Can you work these out from the model? Positions are in its coordinate system, mm. Face numbers are marked on the shaded views. A direction names the side the tool comes from. Give positions to 0.01 mm unless a question says otherwise; leave off trailing zeros. Loops run counter-clockwise (first coordinate to the right, second up) from the corner with the lowest first, then second, coordinate; pieces in that order, holes last. Notation, with made-up numbers: (-7.75, 76) -> (27.25, 76) arc R17 ccw to (27.25, 102) -> close; hole circle Ø10 at (56.25, 46.25). An arc over 180 degrees is marked (long way). One line per question, with ' | ' between items.
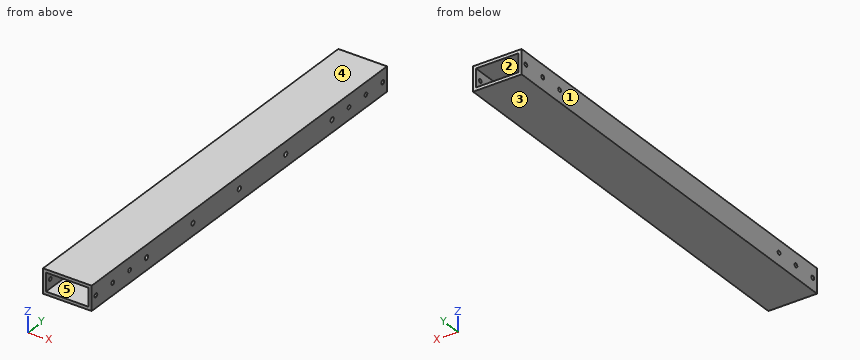
from build123d import *

# Parameters (mm, degrees)
SKETCH1_W           = 50.8
SKETCH1_H           = 25.4
SKETCH1_W_2         = 44.45
SKETCH1_H_2         = 19.05
BOSS_EXTRUDE1_DEPTH = 444.5
CUT_EXTRUDE1_REACH  = 412.536
SKETCH2_R           = 2.0828
SKETCH3_R           = 2.4257
CUT_EXTRUDE2_DEPTH  = 3.175


with BuildPart() as part:
    # Sketch1 → Boss-Extrude1 (new body)
    with BuildSketch(Plane(origin=(0, 0, 0), x_dir=(1, 0, 0), z_dir=(0, 1, 0))):
        with Locations((25.4, 12.7)):
            Rectangle(SKETCH1_W, SKETCH1_H)
        with Locations((25.4, 12.7)):
            Rectangle(SKETCH1_W_2, SKETCH1_H_2, mode=Mode.SUBTRACT)
    extrude(amount=BOSS_EXTRUDE1_DEPTH)

    # Cut-Extrude1: up to this face of the body (flat: up to its plane)
    cut_extrude1_end = Plane(part.part.faces().sort_by_distance((0, 222.25, -12.7))[0])
    # Sketch2 → Cut-Extrude1 (cut, up to the picked face)
    with BuildSketch(Plane(origin=(50.8, 398.917681448, 57.205629331), x_dir=(0, 0, 1), z_dir=(1, 0, 0)), mode=Mode.PRIVATE) as cut_extrude1_sk1:
        with Locations(Location((-69.905629331, -39.232318552, 0), (0, 0, 180))):
            Circle(SKETCH2_R)
    cut_extrude1_tool1 = split(extrude(cut_extrude1_sk1.sketch, amount=-CUT_EXTRUDE1_REACH, mode=Mode.PRIVATE), bisect_by=cut_extrude1_end, keep=Keep.BOTH, mode=Mode.PRIVATE)
    # Sketch2 → Cut-Extrude1 (cut, up to the picked face)
    with BuildSketch(Plane(origin=(50.8, 398.917681448, 57.205629331), x_dir=(0, 0, 1), z_dir=(1, 0, 0)), mode=Mode.PRIVATE) as cut_extrude1_sk2:
        with Locations(Location((-69.905629331, -13.832318552, 0), (0, 0, 180))):
            Circle(SKETCH2_R)
    cut_extrude1_tool2 = split(extrude(cut_extrude1_sk2.sketch, amount=-CUT_EXTRUDE1_REACH, mode=Mode.PRIVATE), bisect_by=cut_extrude1_end, keep=Keep.BOTH, mode=Mode.PRIVATE)
    # Sketch2 → Cut-Extrude1 (cut, up to the picked face)
    with BuildSketch(Plane(origin=(50.8, 398.917681448, 57.205629331), x_dir=(0, 0, 1), z_dir=(1, 0, 0)), mode=Mode.PRIVATE) as cut_extrude1_sk3:
        with Locations(Location((-69.905629331, 11.567681448, 0), (0, 0, 180))):
            Circle(SKETCH2_R)
    cut_extrude1_tool3 = split(extrude(cut_extrude1_sk3.sketch, amount=-CUT_EXTRUDE1_REACH, mode=Mode.PRIVATE), bisect_by=cut_extrude1_end, keep=Keep.BOTH, mode=Mode.PRIVATE)
    # Sketch2 → Cut-Extrude1 (cut, up to the picked face)
    with BuildSketch(Plane(origin=(50.8, 398.917681448, 57.205629331), x_dir=(0, 0, 1), z_dir=(1, 0, 0)), mode=Mode.PRIVATE) as cut_extrude1_sk4:
        with Locations(Location((-69.905629331, 341.767681448, 0), (0, 0, 180))):
            Circle(SKETCH2_R)
    cut_extrude1_tool4 = split(extrude(cut_extrude1_sk4.sketch, amount=-CUT_EXTRUDE1_REACH, mode=Mode.PRIVATE), bisect_by=cut_extrude1_end, keep=Keep.BOTH, mode=Mode.PRIVATE)
    # Sketch2 → Cut-Extrude1 (cut, up to the picked face)
    with BuildSketch(Plane(origin=(50.8, 398.917681448, 57.205629331), x_dir=(0, 0, 1), z_dir=(1, 0, 0)), mode=Mode.PRIVATE) as cut_extrude1_sk5:
        with Locations(Location((-69.905629331, 367.167681448, 0), (0, 0, 180))):
            Circle(SKETCH2_R)
    cut_extrude1_tool5 = split(extrude(cut_extrude1_sk5.sketch, amount=-CUT_EXTRUDE1_REACH, mode=Mode.PRIVATE), bisect_by=cut_extrude1_end, keep=Keep.BOTH, mode=Mode.PRIVATE)
    # Sketch2 → Cut-Extrude1 (cut, up to the picked face)
    with BuildSketch(Plane(origin=(50.8, 398.917681448, 57.205629331), x_dir=(0, 0, 1), z_dir=(1, 0, 0)), mode=Mode.PRIVATE) as cut_extrude1_sk6:
        with Locations(Location((-69.905629331, 392.567681448, 0), (0, 0, 180))):
            Circle(SKETCH2_R)
    cut_extrude1_tool6 = split(extrude(cut_extrude1_sk6.sketch, amount=-CUT_EXTRUDE1_REACH, mode=Mode.PRIVATE), bisect_by=cut_extrude1_end, keep=Keep.BOTH, mode=Mode.PRIVATE)
    add(cut_extrude1_tool1.solids().sort_by(Axis((50.8, 438.15, -12.7), (-1, 0, 0)))[0], mode=Mode.SUBTRACT)
    add(cut_extrude1_tool2.solids().sort_by(Axis((50.8, 412.75, -12.7), (-1, 0, 0)))[0], mode=Mode.SUBTRACT)
    add(cut_extrude1_tool3.solids().sort_by(Axis((50.8, 387.35, -12.7), (-1, 0, 0)))[0], mode=Mode.SUBTRACT)
    add(cut_extrude1_tool4.solids().sort_by(Axis((50.8, 57.15, -12.7), (-1, 0, 0)))[0], mode=Mode.SUBTRACT)
    add(cut_extrude1_tool5.solids().sort_by(Axis((50.8, 31.75, -12.7), (-1, 0, 0)))[0], mode=Mode.SUBTRACT)
    add(cut_extrude1_tool6.solids().sort_by(Axis((50.8, 6.35, -12.7), (-1, 0, 0)))[0], mode=Mode.SUBTRACT)

    # Sketch3 → Cut-Extrude2 (cut)
    with BuildSketch(Plane(origin=(50.8, 398.917681448, 57.205629331), x_dir=(0, 0, 1), z_dir=(1, 0, 0))):
        with Locations(Location((-69.905629331, 36.967681448, 0), (0, 0, 180))):
            Circle(SKETCH3_R)
        with Locations(Location((-69.905629331, 106.817681448, 0), (0, 0, 180))):
            Circle(SKETCH3_R)
        with Locations(Location((-69.905629331, 176.667681448, 0), (0, 0, 180))):
            Circle(SKETCH3_R)
        with Locations(Location((-69.905629331, 246.517681448, 0), (0, 0, 180))):
            Circle(SKETCH3_R)
        with Locations(Location((-69.905629331, 316.367681448, 0), (0, 0, 180))):
            Circle(SKETCH3_R)
    extrude(amount=-CUT_EXTRUDE2_DEPTH, mode=Mode.SUBTRACT)


solid = part.part
Q1. If we section it at A-A (x = 31): Write out the boundary of the cut face in (y, z) (3 decimals), plus the area to 3 significant figures.
Entries:
outline: (0, -25.4) -> (444.5, -25.4) -> (444.5, -22.225) -> (0, -22.225) -> close; (0, -3.175) -> (444.5, -3.175) -> (444.5, 0) -> (0, 0) -> close | area: 2,820 mm²
Q2. If we mould it in two halves opening along Z, with no side actions, what happens to the marked faces 1, 2 and 3? For each: pulls with the +Z half, pulls with the -Z half, needs draft (parallel to the pull), parting line crosses it, or undercut.
Entries:
face 1: needs draft | face 2: undercut | face 3: pulls with the -Z half
Q3. On a 3-axis mill with a long thin cutter (end or side, diameter ignored), from which of +Z, -Z, +X, -X, +Y, -Y can I reach the whole of each face in a straight line? I mean the marked faces 4 and 5. Say none if no direction works.
Entries:
face 4: +Z, +X, -X, +Y, -Y | face 5: +Y, -Y
Q4. For pin 1 Ø3.5 at (y, z) = (31.75, -12.7) entering from -X, with a flat end and sliding along its axis, tell me the tip position at first contact or that it passes through.
Entries:
pin 1: through
Q5. If we section it at B-B (y = 324.5): Write out the boundary of the cut face in (x, z) (3 decimals).
Entries:
outline: (0, -25.4) -> (50.8, -25.4) -> (50.8, 0) -> (0, 0) -> close; hole (3.175, -22.225) -> (47.625, -22.225) -> (47.625, -3.175) -> (3.175, -3.175) -> close
Q6. If I drill on probe 1 along X at (y, z) = (155.5, -5) (3 decimals); probe 2 along Z at (x, y) = (27.5, 307) (3 decimals); probe 3 along Z at (x, y) = (49, 152), over which ranges is the centre line in solid material (lowest first)? Write a range as from..to.
Entries:
probe 1: 0..3.175, 47.625..50.8 | probe 2: -25.4..-22.225, -3.175..0 | probe 3: -25.4..-15.09, -10.31..0
